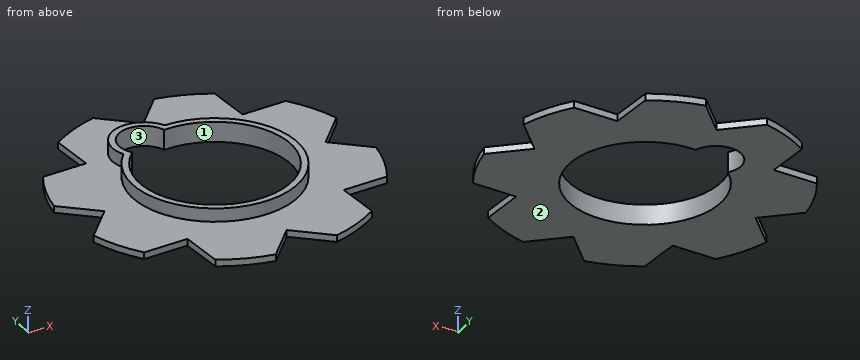
```python
from build123d import *

# Parameters (mm, degrees)
BOSS_EXTRUDE1_DEPTH = 2
BOSS_EXTRUDE2_DEPTH = 4


with BuildPart() as part:
    # Sketch1 → Boss-Extrude1 (new body)
    with BuildSketch(Plane.XY):
        with BuildLine():
            Line((-6.539551855, -44.572825371), (2.326465122, -34.421469464))
            Line((2.326465122, -34.421469464), (12.47782103, -43.287486441))
            ThreePointArc((12.47782103, -43.287486441), (20.007292075, -40.363483049), (26.893585614, -36.141908539))
            Line((26.893585614, -36.141908539), (25.98471374, -22.694595212))
            Line((25.98471374, -22.694595212), (39.432027067, -21.785723338))
            ThreePointArc((39.432027067, -21.785723338), (42.688584475, -14.394000677), (44.572825371, -6.539551855))
            Line((44.572825371, -6.539551855), (34.421469464, 2.326465122))
            Line((34.421469464, 2.326465122), (43.287486441, 12.47782103))
            ThreePointArc((43.287486441, 12.47782103), (40.363483049, 20.007292075), (36.141908539, 26.893585614))
            Line((36.141908539, 26.893585614), (22.694595212, 25.98471374))
            Line((22.694595212, 25.98471374), (21.785723338, 39.432027067))
            ThreePointArc((21.785723338, 39.432027067), (14.394000677, 42.688584475), (6.539551855, 44.572825371))
            Line((6.539551855, 44.572825371), (-2.326465122, 34.421469464))
            Line((-2.326465122, 34.421469464), (-12.47782103, 43.287486441))
            ThreePointArc((-12.47782103, 43.287486441), (-20.007292075, 40.363483049), (-26.893585614, 36.141908539))
            Line((-26.893585614, 36.141908539), (-25.98471374, 22.694595212))
            Line((-25.98471374, 22.694595212), (-39.432027067, 21.785723338))
            ThreePointArc((-39.432027067, 21.785723338), (-42.688584475, 14.394000677), (-44.572825371, 6.539551855))
            Line((-44.572825371, 6.539551855), (-34.421469464, -2.326465122))
            Line((-34.421469464, -2.326465122), (-43.287486441, -12.47782103))
            ThreePointArc((-43.287486441, -12.47782103), (-40.363483049, -20.007292075), (-36.141908539, -26.893585614))
            Line((-36.141908539, -26.893585614), (-22.694595212, -25.98471374))
            Line((-22.694595212, -25.98471374), (-21.785723338, -39.432027067))
            ThreePointArc((-21.785723338, -39.432027067), (-14.394000677, -42.688584475), (-6.539551855, -44.572825371))
        make_face()
        with BuildLine():
            ThreePointArc((-16.063195097, 15.755118637), (9.992543212, -20.159342255), (-2.811608747, 22.323638956))
            ThreePointArc((-2.811608747, 22.323638956), (-13.323390949, 26.879123007), (-16.063195097, 15.755118637))
        make_face(mode=Mode.SUBTRACT)
    extrude(amount=BOSS_EXTRUDE1_DEPTH)

    # Sketch2 → Boss-Extrude2 (add)
    with BuildSketch(Plane.XY.offset(2)):
        with BuildLine():
            ThreePointArc((-1.518157826, 24.452917961), (-14.211617012, 28.671064541), (-18.540947435, 16.015095011))
            ThreePointArc((-18.540947435, 16.015095011), (10.880769275, -21.951283789), (-1.518157826, 24.452917961))
        make_face()
        with BuildLine():
            ThreePointArc((-16.063195097, 15.755118637), (9.992543212, -20.159342255), (-2.811608747, 22.323638956))
            ThreePointArc((-2.811608747, 22.323638956), (-13.323390949, 26.879123007), (-16.063195097, 15.755118637))
        make_face(mode=Mode.SUBTRACT)
    extrude(amount=BOSS_EXTRUDE2_DEPTH)


solid = part.part
```
Part model, mm, in its own coordinate system. Face numbers are marked on the shaded views. Give positions to 0.01 mm unless a question says otherwise; leave off trailing zeros. Write each loop counter-clockwise with the first axis right and the second up, starting at its lowest first coordinate (ties: lowest second). Pieces come first, ordered by that corner, then holes. Notation, with made-up numbers: (39, 10) -> (72, 10) arc R16 cw to (72, 27) -> close; hole circle Ø10 at (1, 67.25). An arc over 180 degrees is marked (long way). Put each result on its own line as item: value. Start each with the question number.
Item 1: Pull direction Y, two halves, no side cores. Call the marked faces 1, 2 and 3: pulls with the +Y half, pulls with the -Y half, needs draft (parallel to the pull), parting line crosses it, or undercut.
Item 2: Wall check: L1, parallel to Y at x = 0, z = 3.05; L2, parallel to Z at x = 3, y = -26; L3, parallel to X at y = -16.5, z = 4.25. Give the ranges that are in metal, low to high. Write a range as [from, to].
Item 3: Pin check, flat tips, straight feed: pin 1 Ø3 at (y, z) = (6.5, 2) entering from +X; pin 2 Ø2 at (x, y) = (-28, -27.5) entering from -Z; pin 3 Ø2 at (y, z) = (-16, 2) entering from +X. Stop position of each tip, or through.
Item 4: Cut at A-A (x = -5). List the corners of the cut face in (y, z).
Item 5: Cut at D-D (x = 32.5). List the corners of the cut face in (y, z), then the cut area to 3 significant figures.
Item 6: Cut at B-B (y = -5). List the corners of the cut face in (x, z).
Item 7: Cut at C-C (z = 4.25). List the corners of the cut face in (x, y).
Answer list:
1. face 1: undercut
1. face 2: needs draft
1. face 3: undercut
2. L1: y = [-24.5, -22.5], [22.5, 24.5]
2. L2: z = [0, 2]
2. L3: x = [-18.11, -15.3], [15.3, 18.11]
3. pin 1: stops at x = 39.38
3. pin 2: passes through
3. pin 3: stops at x = 42.48
4. outline: (-42.81, 0) -> (-21.94, 0) -> (-21.94, 6) -> (-23.98, 6) -> (-23.98, 2) -> (-42.81, 2) -> close; (25.76, 0) -> (36.76, 0) -> (36.76, 2) -> (28.24, 2) -> (28.24, 6) -> (25.76, 6) -> close
5. outline: (-22.25, 0) -> (26.65, 0) -> (26.65, 2) -> (-22.25, 2) -> close
5. area: 97.8 mm2
6. outline: (-36.76, 0) -> (-21.94, 0) -> (-21.94, 6) -> (-23.98, 6) -> (-23.98, 2) -> (-36.76, 2) -> close; (21.94, 0) -> (42.81, 0) -> (42.81, 2) -> (23.98, 2) -> (23.98, 6) -> (21.94, 6) -> close
7. outline: (-18.54, 16.02) arc R24.5 ccw (long way) to (-1.52, 24.45) arc R9.5 ccw to start; hole (-16.06, 15.76) arc R22.5 ccw (long way) to (-2.81, 22.32) arc R7.5 ccw (long way) to start
